Autodesk Inventor part; units mm, degrees
ref_plane "Work Plane1" through (-85, 10, -35) normal (-1, 0, 0) x (0, 0, 1)
ref_plane "YZ Plane" through (0, 0, 0) normal (1, 0, 0) x (0, 1, 0)
ref_plane "XZ Plane" through (0, 0, 0) normal (0, 1, 0) x (-1, 0, 0)
sketch "Sketch1" plane through (0, 0, 0) normal (0, 1, 0) x (-1, 0, 0)
  line L0 (0, 0) -> (105, 0)
  line L1 (105, 0) -> (105, -35)
  line L2 (105, -35) -> (0, -35)
  line L3 (0, -35) -> (0, 0)
  dimension "d0" = 35
  dimension "d1" = 105
extrude "Extrusion1" add sketch "Sketch1" along normal blind 10
sketch "Sketch2" plane through (0, 10, 0) normal (0, 1, 0) x (1, 0, 0)
  circle A0 centre (-20, 17.5) radius 11.25
  line L0 (0, 35) -> (-105, 35)
  line L1 (-105, 35) -> (-105, 0)
  point P0 (0, 0)
  dimension "d4" = 22.5
  dimension "d5" = 17.5
  dimension "d6" = 85
extrude "Extrusion2" cut sketch "Sketch2" against normal blind 5
sketch "Sketch3" plane through (0, 0, 0) normal (0, -1, 0) x (1, 0, 0)
  circle A0 centre (-20, -17.5) radius 11.25 construction
  point P0 (0, 0)
hole "Hole1" at (-20, 0, -17.5) direction (0, 1, 0) diameter 4 depth 8 tip angle 118 counterbore diameter 6.5 counterbore depth 1
sketch "Sketch4" plane through (0, 0, 0) normal (0, -1, 0) x (1, 0, 0)
  line L0 (-105, -35) -> (0, -35)
  line L1 (-105, -35) -> (-85, -35)
  line L2 (-85, -35) -> (-85, 0)
  line L3 (-85, 0) -> (-105, 0)
  line L4 (-105, 0) -> (-105, -35)
  point P0 (0, 0)
  dimension "d16" = 20
extrude "Extrusion3" add sketch "Sketch4" along normal blind 40
sketch "Sketch5" plane through (-105, 10, 0) normal (0, 0, 1) x (1, 0, 0)
  line L0 (20, -50) -> (0, -50)
  line L1 (8.7445, -50) -> (20, -19.0668)
  line L2 (20, -10) -> (20, -50)
  line L3 (20, -50) -> (8.7445, -50)
  line L4 (20, -50) -> (20, -19.0668)
  point P0 (105, -10)
extrude "Extrusion4" cut sketch "Sketch5" against normal blind 42
ref_plane "Work Plane1" through (-85, 10, -35) normal (-1, 0, 0) x (0, 0, 1)
sketch "Sketch6" plane through (-85, 10, -35) normal (-1, 0, 0) x (0, 0, 1)
  circle A0 centre (27, -42) radius 4.25
  line L0 (35, -50) -> (35, -19.0668)
  line L1 (0, -50) -> (35, -50)
  circle A1 centre (8, -27.0668) radius 4.25
  line L2 (35, -19.0668) -> (0, -19.0668)
  line L3 (0, -19.0668) -> (0, -50)
  point P0 (35, -10)
  dimension "d22" = 8.5
  dimension "d23" = 8
  dimension "d24" = 8
  dimension "d25" = 8.5
  dimension "d26" = 8
  dimension "d27" = 8
extrude "Extrusion5" cut sketch "Sketch6" along normal blind 11 contours A0 | A1
sketch "Sketch7" plane through (-96, -32, -8) normal (1, 0, 0) x (0, 0, -1)
  point P0 (-8, 32)
  point P1 (0, 0)
hole "Hole2" at (-96, -32, -8) direction (-1, 0, 0) diameter 4.5 depth 10 tip angle 118
sketch "Sketch8" plane through (-96, -17.0668, -27) normal (1, 0, 0) x (0, 0, -1)
  point P0 (-27, 17.0668)
  point P1 (0, 0)
hole "Hole3" at (-96, -17.0668, -27) direction (-1, 0, 0) diameter 4.5 depth 10 tip angle 118
fillet "Fillet1" radius 4 1 edges at (-85, 0, -17.5)
fillet "Fillet2" radius 15 1 edges at (0, 5, 0)
fillet "Fillet3" radius 15 1 edges at (0, 5, -35)
properties part number "Large Bracket (RHS)"
The model under review builds one solid part; all positions refer to its coordinate system, in mm. A direction names the side the tool comes from. Round coordinates to 2 decimals unless told otherwise and drop trailing zeros. Write each loop counter-clockwise with the first axis right and the second up, starting at its lowest first coordinate (ties: lowest second). Pieces come first, ordered by that corner, then holes. Notation, with made-up numbers: M -14.5,14 L 32.5,14 A18 cw 32.5,37 Z; hole C 39,33.5 d6. An arc over 180 degrees is marked long. Use CSV: the item, a comma, the result in double quotes. Start each with the question number.
(1) We need section B-B, the plane x = -20. State the section outline as (y, z) points, then the cut area to 3 significant figures.
(2) For line 1 along Z through (x, y) = (-20, 0.6); line 2 along Z through (x, y) = (-20, 6.35); line 3 along Y through (x, z) = (-101.5, -8), list the stretches that pass through material, from the lowest coordinate up.
(3) Clearance check with flat-ended pins moving along their axes: P1, Ø5, axis at x = -20, z = -19, coming from the -Y side; P2, Ø10.5, axis at x = -20, z = -17.5, coming from the +Y side; P3, Ø3, axis at y = -27.5, z = -29.5, coming from the +X side; P4, Ø13.5, axis at y = -32, z = -8, coming from the -X side. State where each tip first meets the part, or that it passes through.
(4) We need section A-A, the plane z = -17.5. State the section outline as (x, y) points.
(5) We need section C-C, the plane y = -32. State the section outline as (x, z) points.
(6) The part is to be moulded in two halves that separate along Z. For faces 4 (the face through (-92.183, -12.918, -27.921)), 5 (the face through (-74, 2, -35)), 6 (the face through (-76, 2, 0)), 7 (the face through (-83.797, -1.141, -17.255)), say which applies: +Z half, -Z half, draft (parallel to the pull), parting line (faces both ways), or undercut.
(7) Tool access review of faces 1 (the face through (-20, 5, -15)), 2 (the face through (-85, -6, -18)), 3 (the face through (-96, -19, -25)): name each direction out of +Z, -Z, +X, -X, +Y, -Y from which nothing blocks a thin tool from reaching the whole face with its end or side.
(8) We need section D-D, the plane z = -27. State the section outline as (x, y) points, then the cut area to 3 significant figures.
Findings:
1,outline,"M 0,-35 L 10,-35 L 10,-28.75 L 5,-28.75 L 5,-19.5 L 1,-19.5 L 1,-20.75 L 0,-20.75 Z; M 0,-14.25 L 1,-14.25 L 1,-15.5 L 5,-15.5 L 5,-6.25 L 10,-6.25 L 10,0 L 0,0 Z"
1,area,"215 mm^2"
2,line 1,"-35 to -20.75, -14.25 to 0"
2,line 2,"-35 to -28.75, -6.25 to 0"
2,line 3,"-40 to -34.25, -29.75 to 10"
3,P1,"y = 0"
3,P2,"y = 5"
3,P3,"x = -91.16"
3,P4,"x = -105"
4,outline,"M -105,-40 L -96.26,-40 L -85,-9.07 L -85,-4 A4 cw -81,0 L -23.25,0 L -23.25,1 L -22,1 L -22,5 L -31.25,5 L -31.25,10 L -105,10 Z; M -18,1 L -16.75,1 L -16.75,0 L 0,0 L 0,10 L -8.75,10 L -8.75,5 L -18,5 Z"
5,outline,"M -105,-35 L -93.34,-35 L -93.34,-12.25 L -96,-12.25 L -96,-10.25 L -105,-10.25 Z; M -105,-5.75 L -96,-5.75 L -96,-3.75 L -93.34,-3.75 L -93.34,0 L -105,0 Z"
6,face 4,"undercut"
6,face 5,"-Z half"
6,face 6,"+Z half"
6,face 7,"draft"
7,face 1,"+Y"
7,face 2,"+Z, -Z, +X, -Y"
7,face 3,"+X"
8,outline,"M -105,-40 L -96.26,-40 L -89.46,-21.32 L -96,-21.32 L -96,-19.32 L -105,-19.32 Z; M -105,-14.82 L -96,-14.82 L -96,-12.82 L -86.36,-12.82 L -85,-9.07 L -85,-4 A4 cw -81,0 L -1.73,0 L -1.73,10 L -13.97,10 L -13.97,5 L -26.03,5 L -26.03,10 L -105,10 Z"
8,area,"1,490 mm^2"
